```python
from build123d import *

# Parameters (mm, degrees)
SKETCH1_W           = 60
SKETCH1_H           = 45
BOSS_EXTRUDE1_DEPTH = 2.032
FILLET1_R           = 5
SKETCH2_W           = 41
SKETCH2_H           = 21
CUT_EXTRUDE1_DEPTH  = 3.032
FILLET2_R           = 0.5
CUT_EXTRUDE2_DEPTH  = 3.032
SKETCH4_R           = 1.6
CUT_EXTRUDE3_DEPTH  = 3.032
CUT_EXTRUDE4_DEPTH  = 3.032
FILLET3_R           = 0.5


with BuildPart() as part:
    # Sketch1 → Boss-Extrude1 (new body)
    with BuildSketch(Plane.XY):
        Rectangle(SKETCH1_W, SKETCH1_H)
    extrude(amount=BOSS_EXTRUDE1_DEPTH)

    # Fillet1
    fillet1_edges = [part.edges().sort_by_distance(p)[0] for p in [
        (30, -22.5, 1.016),
        (-30, -22.5, 1.016),
        (-30, 22.5, 1.016),
        (30, 22.5, 1.016),
    ]]
    fillet(fillet1_edges, radius=FILLET1_R)

    # Sketch2 → Cut-Extrude1 (cut, through all)
    with BuildSketch(Plane.XY.offset(2.032)):
        with Locations((0, 7.5)):
            Rectangle(SKETCH2_W, SKETCH2_H)
    extrude(amount=-CUT_EXTRUDE1_DEPTH, mode=Mode.SUBTRACT)

    # Fillet2
    fillet2_edges = [part.edges().sort_by_distance(p)[0] for p in [
        (20.5, 18, 1.016),
        (20.5, -3, 1.016),
        (-20.5, -3, 1.016),
        (-20.5, 18, 1.016),
    ]]
    fillet(fillet2_edges, radius=FILLET2_R)

    # Sketch3 → Cut-Extrude2 (cut, through all)
    with BuildSketch(Plane.XY.offset(2.032)):
        with BuildLine():
            Line((-23.4, 3), (-23.4, 2))
            ThreePointArc((-23.4, 2), (-25, 0.4), (-26.6, 2))
            Line((-26.6, 2), (-26.6, 3))
            ThreePointArc((-26.6, 3), (-25, 4.6), (-23.4, 3))
        make_face()
        with BuildLine():
            Line((-23.4, 12), (-23.4, 13))
            ThreePointArc((-23.4, 13), (-25, 14.6), (-26.6, 13))
            Line((-26.6, 13), (-26.6, 12))
            ThreePointArc((-26.6, 12), (-25, 10.4), (-23.4, 12))
        make_face()
        with BuildLine():
            Line((23.4, 3), (23.4, 2))
            ThreePointArc((23.4, 2), (25, 0.4), (26.6, 2))
            Line((26.6, 2), (26.6, 3))
            ThreePointArc((26.6, 3), (25, 4.6), (23.4, 3))
        make_face()
        with BuildLine():
            Line((23.4, 12), (23.4, 13))
            ThreePointArc((23.4, 13), (25, 14.6), (26.6, 13))
            Line((26.6, 13), (26.6, 12))
            ThreePointArc((26.6, 12), (25, 10.4), (23.4, 12))
        make_face()
    extrude(amount=-CUT_EXTRUDE2_DEPTH, mode=Mode.SUBTRACT)

    # Sketch4 → Cut-Extrude3 (cut, through all)
    with BuildSketch(Plane.XY.offset(2.032)):
        with Locations((-15, -15)):
            Circle(SKETCH4_R)
        with Locations((15, -15)):
            Circle(SKETCH4_R)
        with Locations((10, -17.5)):
            Circle(SKETCH4_R)
        with Locations((-10, -17.5)):
            Circle(SKETCH4_R)
        with Locations((20, -17.5)):
            Circle(SKETCH4_R)
        with Locations((-20, -17.5)):
            Circle(SKETCH4_R)
        with BuildLine():
            Line((1.6, -15), (1.6, -17.5))
            ThreePointArc((1.6, -17.5), (0, -19.1), (-1.6, -17.5))
            Line((-1.6, -17.5), (-1.6, -15))
            ThreePointArc((-1.6, -15), (0, -13.4), (1.6, -15))
        make_face()
    extrude(amount=-CUT_EXTRUDE3_DEPTH, mode=Mode.SUBTRACT)

    # Sketch5 → Cut-Extrude4 (cut, through all)
    with BuildSketch(Plane.XY.offset(2.032)):
        with BuildLine():
            Line((-21, -3), (21, -3))
            ThreePointArc((21, -3), (21.353553391, -2.853553391), (21.5, -2.5))
            Line((21.5, -2.5), (21.5, 3))
            Line((21.5, 3), (23.4, 3))
            ThreePointArc((23.4, 3), (24.53137085, 3.46862915), (25, 4.6))
            Line((25, 4.6), (25, 10.4))
            ThreePointArc((25, 10.4), (24.53137085, 11.53137085), (23.4, 12))
            Line((23.4, 12), (21.5, 12))
            Line((21.5, 12), (21.5, 17.5))
            ThreePointArc((21.5, 17.5), (21.353553391, 17.853553391), (21, 18))
            Line((21, 18), (-21, 18))
            ThreePointArc((-21, 18), (-21.353553391, 17.853553391), (-21.5, 17.5))
            Line((-21.5, 17.5), (-21.5, 12))
            Line((-21.5, 12), (-23.4, 12))
            ThreePointArc((-23.4, 12), (-24.53137085, 11.53137085), (-25, 10.4))
            Line((-25, 10.4), (-25, 4.6))
            ThreePointArc((-25, 4.6), (-24.53137085, 3.46862915), (-23.4, 3))
            Line((-23.4, 3), (-21.5, 3))
            Line((-21.5, 3), (-21.5, -2.5))
            ThreePointArc((-21.5, -2.5), (-21.353553391, -2.853553391), (-21, -3))
        make_face()
    extrude(amount=-CUT_EXTRUDE4_DEPTH, mode=Mode.SUBTRACT)

    # Fillet3
    fillet3_edges = [part.edges().sort_by_distance(p)[0] for p in [
        (23.4, 3, 1.016),
        (23.4, 12, 1.016),
        (-21.5, 3, 1.016),
        (-25, 4.6, 1.016),
        (-25, 10.4, 1.016),
        (-21.5, 12, 1.016),
        (21.5, 12, 1.016),
        (25, 10.4, 1.016),
        (25, 4.6, 1.016),
        (21.5, 3, 1.016),
        (-23.4, 3, 1.016),
        (-23.4, 12, 1.016),
    ]]
    fillet(fillet3_edges, radius=FILLET3_R)


solid = part.part
```
The listing builds one solid part. Answer for the finished solid, in the listing's coordinates (mm). A direction names the side the tool comes from. Coordinates: 2 decimals unless noted, no trailing zeros. Write each loop counter-clockwise with the first axis right and the second up, starting at its lowest first coordinate (ties: lowest second). Pieces come first, ordered by that corner, then holes. Notation, with made-up numbers: (61, 54.5) - (90, 54.5) arc R25 cw to (90, 69.5) - close; hole circle Ø11 at (-31, 62.5). An arc over 180 degrees is marked (long way). One line per item, written item: value.
1) For a pull along X with two mould halves and no side action, classify faces 3 (the cylindrical face through (28.57, 21, 1.03)), 4 (the cylindrical face through (-26.268, 3.976, 1.03)), 5 (the flat face through (21.5, 0, 1)), 6 (the cylindrical face through (-28.57, 21, 1.03)) as pulls with the +X half, pulls with the -X half, needs draft (parallel to the pull), parting line crosses it, or undercut.
Geometry check:
face 3: pulls with the +X half
face 4: undercut
face 5: undercut
face 6: pulls with the -X half
2) A tool of negligible diameter and unlimited length cuts with its end or side. For faces 1 (the cylindrical face through (26.268, 3.976, 1.03)), 2 (the flat face through (0, -5, 2.032)), from which of +Z, -Z, +X, -X, +Y, -Y can it reach the whole face along a straight path? Write none if from no direction.
Geometry check:
face 1: +Z, -Z
face 2: +Z, +X, -X, +Y, -Y
3) Find section A-A (x = 10). Give the vertices of the cut face in (y, z).
Geometry check:
outline: (-22.5, 0) - (-19.1, 0) - (-19.1, 2.03) - (-22.5, 2.03) - close; (-15.9, 0) - (-3, 0) - (-3, 2.03) - (-15.9, 2.03) - close; (18, 0) - (22.5, 0) - (22.5, 2.03) - (18, 2.03) - close
4) Consider line 1 along Y through (x, z) = (-20, 0.7); line 2 along Y through (x, z) = (15, 1.2); line 3 along Y through (x, z) = (-5, 0.1). Determine where each line is inside the solid, lowest interval first. Write a range as from..to.
Geometry check:
line 1: y = -22.5..-19.1, -15.9..-3, 18..22.5
line 2: y = -22.5..-16.6, -13.4..-3, 18..22.5
line 3: y = -22.5..-3, 18..22.5
5) This flat-tipped pin is pushed along its axis until it touches: pin 1 Ø2.5 at (x, y) = (-15, -15) entering from -Z. Where does it stop, or does it pass through?
Geometry check:
pin 1: passes through
6) Find section B-B (z = 1.6). Count the separate pieces of the cut face and the enclosed holes in it, and give its area (3 significant figures).
Geometry check:
separate pieces: 1
enclosed holes: 8
area: 1,610 mm2
